Here's the drawing with two shaded views (mm, measured from the low corner). I have some questions. A direction names the side the tool comes from. Give positions to 0.01 mm unless a question says otherwise; leave off trailing zeros. Loops run counter-clockwise (first coordinate to the right, second up) from the corner with the lowest first, then second, coordinate; pieces in that order, holes last. Notation, with made-up numbers: (58.5, 36.25) - (100.5, 36.25) arc R26 ccw to (100.5, 69.25) - close; hole circle Ø4 at (58, -38.75). An arc over 180 degrees is marked (long way). Answer as a JSON object with one key per item and string values. Group by question number.
Item 1: Suppose I cut it at B-B on y = 0.7. Write out the boundary of the cut face in (x, z).
Item 2: Please list where these lines run through material, in increasing order: L1, parallel to Y at x = 1.75, z = 4; L2, parallel to Z at x = 14.25, y = 2.5; L3, parallel to X at y = 4.6, z = 1.5.
Item 3: Suppose I cut it at D-D on y = 4.35. Write out the boundary of the cut face in (x, z).
Item 4: Suppose I cut it at C-C on x = 16. Write out the boundary of the cut face in (y, z).
Item 5: Suppose I cut it at A-A on z = 1.5. Write out the boundary of the cut face in (x, y), and give its area (4 significant figures).
Item 6: Will these pins go through, and if not, where does the flat tip stop? pin 1 (1.5 mm diameter, centred on y = 3.5, z = 2, fed in from -X); pin 2 (2 mm diameter, centred on x = 8, y = 3, fed in from +Z); pin 3 (2.5 mm diameter, centred on y = 3, z = 2, fed in from +X).
Item 7: Which directions (+Z, -Z, +X, -X, +Y, -Y) give clear straight access to the entire face, cutting with the end or side of a thin tool? Please do the marked faces 1, 2 and 3.
Item 8: Thinking about a two-plate mould opening in Z: for the marked faces 4, 5 and 6, which applies, pulls with the +Z half, pulls with the -Z half, needs draft (parallel to the pull), parting line crosses it, or undercut?
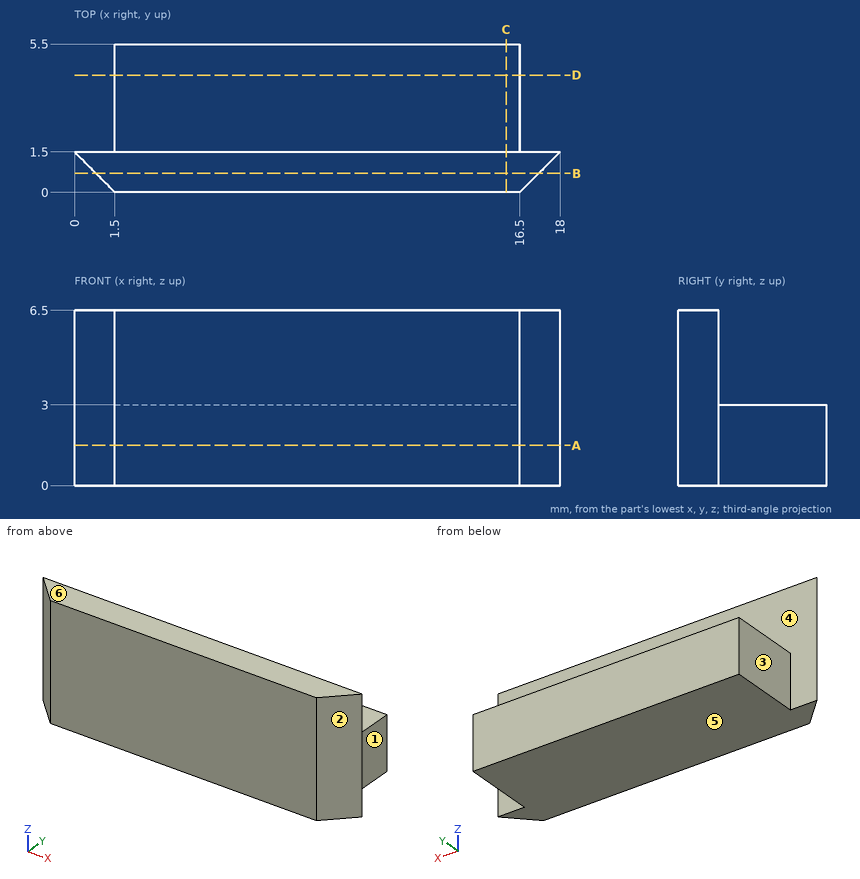
Worked out:
{
 "1": {"outline": "(0.8, 0) - (17.2, 0) - (17.2, 6.5) - (0.8, 6.5) - close"},
 "2": {"L1": "y = 0 to 1.5", "L2": "z = 0 to 3", "L3": "x = 1.5 to 16.5"},
 "3": {"outline": "(1.5, 0) - (16.5, 0) - (16.5, 3) - (1.5, 3) - close"},
 "4": {"outline": "(0, 0) - (5.5, 0) - (5.5, 3) - (1.5, 3) - (1.5, 6.5) - (0, 6.5) - close"},
 "5": {"outline": "(0, 1.5) - (1.5, 0) - (16.5, 0) - (18, 1.5) - (16.5, 1.5) - (16.5, 5.5) - (1.5, 5.5) - (1.5, 1.5) - close", "area": "84.75 mm2"},
 "6": {"pin 1": "stops at x = 1.5", "pin 2": "stops at z = 3", "pin 3": "stops at x = 16.5"},
 "7": {"face 1": "+Z, -Z, +X, +Y", "face 2": "+Z, -Z, +X, -Y", "face 3": "+Z, -Z, -X, +Y"},
 "8": {"face 4": "needs draft", "face 5": "pulls with the -Z half", "face 6": "pulls with the +Z half"}
}
